Input: part model. Units: mm. Frame: model coordinates. A direction names the side the tool comes from. Give positions to 0.01 mm unless a question says otherwise; leave off trailing zeros. Loops run counter-clockwise (first coordinate to the right, second up) from the corner with the lowest first, then second, coordinate; pieces in that order, holes last. Notation, with made-up numbers: M 75,55.25 L 80,55.25 A17 cw 80,81.25 Z; hole C 58,49 d2. An arc over 180 degrees is marked long. Use a Markdown table: item, result. Add a question column.
from build123d import *

# Parameters (mm, degrees)
SALIENTE_EXTRUIR1_DEPTH = 4


with BuildPart() as part:
    # Croquis1 → Saliente-Extruir1 (new body)
    with BuildSketch(Plane.XY):
        with BuildLine():
            Line((0, 23.001027223), (-5, 23.001027223))
            Line((-5, 23.001027223), (-5, 12.001027223))
            ThreePointArc((-5, 12.001027223), (-4.121320344, 9.87970688), (-2, 9.001027223))
            Line((-2, 9.001027223), (7, 9.001027223))
            ThreePointArc((7, 9.001027223), (9.121320344, 9.87970688), (10, 12.001027223))
            Line((10, 12.001027223), (10, 19.001027223))
            Line((10, 19.001027223), (6, 19.001027223))
            Line((6, 19.001027223), (6, 17.501027223))
            Line((6, 17.501027223), (8.5, 17.501027223))
            Line((8.5, 17.501027223), (8.5, 14.501027223))
            Line((8.5, 14.501027223), (-0.5, 14.501027223))
            Line((-0.5, 14.501027223), (-0.5, 17.501027223))
            Line((-0.5, 17.501027223), (2, 17.501027223))
            Line((2, 17.501027223), (2, 19.001027223))
            Line((2, 19.001027223), (0, 19.001027223))
            Line((0, 19.001027223), (0, 23.001027223))
        make_face()
    extrude(amount=SALIENTE_EXTRUIR1_DEPTH)


solid = part.part
1) Reachability of faces 1 (the flat face through (4, 14.501, 2)), 2 (the flat face through (1, 19.001, 2)), 3 (the flat face through (6, 18, 2)) from +Z, -Z, +X, -X, +Y, -Y: full face, straight path, thin tool, end or side. Return the list, or none.
2) Section query B-B, the plane x = 6.25. Return the cut outline in (y, z), and give its area (3 significant figures).
3) Contact query for flat-ended pins moving along their axis: P1, Ø1.2, axis at y = 20, z = 2, coming from the +X side; P2, Ø1.5, axis at x = 0.5, y = 15.5, coming from the -Z side; P3, Ø2, axis at x = 4, z = 2, coming from the +Y side; P4, Ø1, axis at x = 1, z = 1.5, coming from the +Y side. Output: stop coordinate, or through.
4) Ray query, line 1 (Y direction, x = 1, z = 0.3); line 2 (X direction, y = 18, z = 2.85); line 3 (X direction, y = 17, z = 3.65). Return the intervals inside material, ascending. Write a range as [from, to].
5) Section query C-C, the plane y = 18.75. Return the cut outline in (x, z), and give its area (3 significant figures).
6) Section query A-A, the plane z = 2.8. Return the cut outline in (x, y), and give its area (3 significant figures).
7) Section query D-D, the plane x = 9.25. Return the cut outline in (y, z), and give its area (3 significant figures).
Entries:
| question | item | result |
|---|---|---|
| 1 | face 1 | +Z, -Z |
| 1 | face 2 | +Z, -Z, +X, +Y |
| 1 | face 3 | +Z, -Z, +Y |
| 2 | outline | M 9,0 L 14.5,0 L 14.5,4 L 9,4 Z; M 17.5,0 L 19,0 L 19,4 L 17.5,4 Z |
| 2 | area | 28.0 mm² |
| 3 | P1 | stops at x = 0 |
| 3 | P2 | passes through |
| 3 | P3 | stops at y = 14.5 |
| 3 | P4 | stops at y = 19 |
| 4 | line 1 | y = [9, 14.5], [17.5, 19] |
| 4 | line 2 | x = [-5, 2], [6, 10] |
| 4 | line 3 | x = [-5, -0.5], [8.5, 10] |
| 5 | outline | M -5,0 L 2,0 L 2,4 L -5,4 Z; M 6,0 L 10,0 L 10,4 L 6,4 Z |
| 5 | area | 44.0 mm² |
| 6 | outline | M -5,12 A3 ccw -2,9 L 7,9 A3 ccw 10,12 L 10,19 L 6,19 L 6,17.5 L 8.5,17.5 L 8.5,14.5 L -0.5,14.5 L -0.5,17.5 L 2,17.5 L 2,19 L 0,19 L 0,23 L -5,23 Z |
| 6 | area | 133 mm² |
| 7 | outline | M 10.02,0 L 19,0 L 19,4 L 10.02,4 Z |
| 7 | area | 35.9 mm² |
